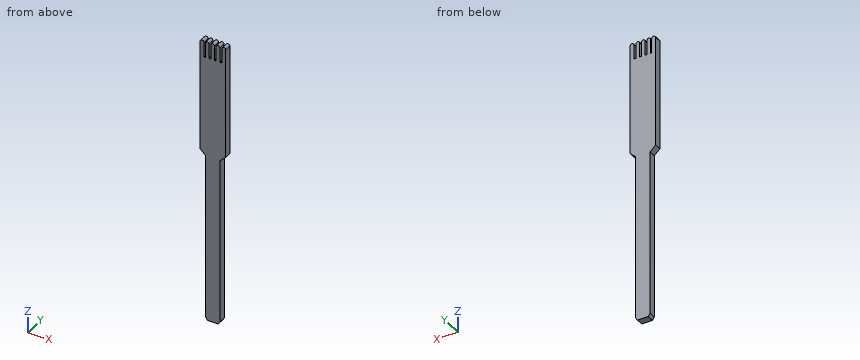
```python
from build123d import *

# Parameters (mm, degrees)
F1_DEPTH = 6.35


with BuildPart() as f1:
    # F0 (on Front) → F1 (new body)
    with BuildSketch(Plane.XZ):
        with BuildLine():
            Line((-8.085411, 13.072304), (-8.085411, -139.327696))
            Line((-8.085411, -139.327696), (-6.365239, -141.902923))
            Line((-6.365239, -141.902923), (3.477706, -141.902923))
            Line((3.477706, -141.902923), (5.168511, -139.327696))
            Line((5.168511, -139.327696), (5.168511, 13.072304))
            Line((5.168511, 13.072304), (10.259341, 17.928839))
            Line((10.259341, 17.928839), (10.259341, 119.528839))
            ThreePointArc((10.259341, 119.528839), (8.576134, 121.212046), (6.892927, 119.528839))
            Line((6.892927, 119.528839), (6.892927, 106.053379))
            Line((6.892927, 106.053379), (4.900902, 106.053379))
            Line((4.900902, 106.053379), (4.900902, 119.528839))
            ThreePointArc((4.900902, 119.528839), (3.201823, 121.227918), (1.502743, 119.528839))
            Line((1.502743, 119.528839), (1.502743, 106.053379))
            Line((1.502743, 106.053379), (0, 106.053379))
            Line((0, 106.053379), (0, 119.528839))
            ThreePointArc((0, 119.528839), (-1.709364, 121.238202), (-3.418728, 119.528839))
            Line((-3.418728, 119.528839), (-3.418728, 106.053379))
            Line((-3.418728, 106.053379), (-5.176397, 106.053379))
            Line((-5.176397, 106.053379), (-5.176397, 119.528839))
            ThreePointArc((-5.176397, 119.528839), (-6.816888, 121.16933), (-8.457379, 119.528839))
            Line((-8.457379, 119.528839), (-8.457379, 106.053379))
            Line((-8.457379, 106.053379), (-9.51198, 106.053379))
            Line((-9.51198, 106.053379), (-9.51198, 119.528839))
            ThreePointArc((-9.51198, 119.528839), (-11.344111, 121.360969), (-13.176241, 119.528839))
            Line((-13.176241, 119.528839), (-13.176241, 17.928839))
            Line((-13.176241, 17.928839), (-8.085411, 13.072304))
        make_face()
    extrude(amount=F1_DEPTH)


solid = f1.part
```
Geometry: final body of the model. Coordinates: model frame, mm. Give positions to 0.01 mm unless a question says otherwise; leave off trailing zeros. Write each loop counter-clockwise with the first axis right and the second up, starting at its lowest first coordinate (ties: lowest second). Pieces come first, ordered by that corner, then holes.
1. Pin query (flat end, axial travel): P1, Ø0.8, axis at x = 0.5, y = -2, coming from the +Z side; P2, Ø1.2, axis at x = -8.5, y = -3.5, coming from the +Z side; P3, Ø3, axis at y = -1.5, z = -73.5, coming from the -X side. Return the tip coordinate at first contact, or that it passes through.
2. Line query: probe 1 along X at (y, z) = (-2.5, 107); probe 2 along X at (y, z) = (-6, 6); probe 3 along Z at (x, y) = (-1.5, -1.25). Output: solid intervals per line, ascending.
3. Section query B-B, the plane z = -11.5. Return loops of the section in (x, y), then the cut area to 3 significant figures.
4. Section query A-A, the plane y = -1.75. Return loops of the section in (x, z).
Computed:
1. P1: stops at z = 106.05
1. P2: stops at z = 120.76
1. P3: stops at x = -8.09
2. probe 1: x = -13.18 to -9.51, -8.46 to -5.18, -3.42 to 0, 1.5 to 4.9, 6.89 to 10.26
2. probe 2: x = -8.09 to 5.17
2. probe 3: z = -141.9 to 121.23
3. outline: (-8.09, -6.35) - (5.17, -6.35) - (5.17, 0) - (-8.09, 0) - close
3. area: 84.2 mm2
4. outline: (-13.18, 17.93) - (-8.09, 13.07) - (-8.09, -139.33) - (-6.37, -141.9) - (3.48, -141.9) - (5.17, -139.33) - (5.17, 13.07) - (10.26, 17.93) - (10.26, 119.53) arc R1.68 ccw to (6.89, 119.53) - (6.89, 106.05) - (4.9, 106.05) - (4.9, 119.53) arc R1.7 ccw to (1.5, 119.53) - (1.5, 106.05) - (0, 106.05) - (0, 119.53) arc R1.71 ccw to (-3.42, 119.53) - (-3.42, 106.05) - (-5.18, 106.05) - (-5.18, 119.53) arc R1.64 ccw to (-8.46, 119.53) - (-8.46, 106.05) - (-9.51, 106.05) - (-9.51, 119.53) arc R1.83 ccw to (-13.18, 119.53) - close
